Drawing for the job (mm, zero at the part's lowest x, y, z). A direction names the side the tool comes from. Give positions to 0.01 mm unless a question says otherwise; leave off trailing zeros. Order: outer loops, then holes, each group sorted by start corner. A loop starts at its lowest first (then second) coordinate and runs counter-clockwise, first axis right, second up. Notation, with made-up numbers: (16.5, 67) -> (47.5, 67) arc R19 cw to (47.5, 94) -> close; hole circle Ø5 at (-31.75, -21.5). An arc over 180 degrees is marked (long way). One line per item, written item: value. Start each with the question number.
(1) Saw through at B-B on y = 12.5. Give the cut face in (x, z).
(2) Which spindle directions (+Z, -Z, +X, -X, +Y, -Y) get a long thin tool onto all of the face, cutting with end or side? Do the marked faces 1 and 2. Say none if no direction does.
(3) Saw through at A-A on z = 2.4. Give the cut face in (x, y) (1 decimal).
(4) Probe line 1 (X direction, y = 4.5, z = 2.2); line 2 (Y direction, x = 1.65, z = 1.5) (1 decimal); line 3 (Y direction, x = 1.8, z = 1.6) (1 decimal). List the from-to ranges inside material, lowest first.
(5) Saw through at C-C on x = 2.75. Give the cut face in (y, z).
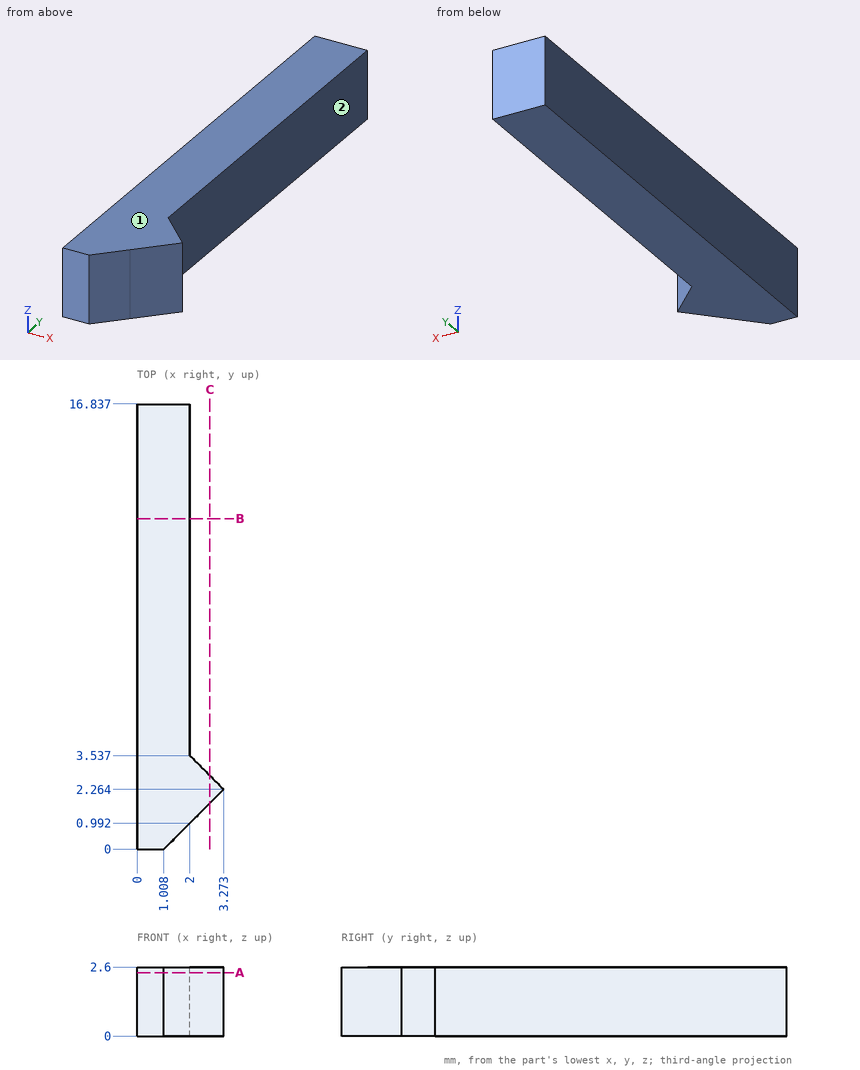
Results below:
1. outline: (0, 0) -> (2, 0) -> (2, 2.6) -> (0, 2.6) -> close
2. face 1: +Z, +X, -X, +Y, -Y
2. face 2: +Z, -Z, +X, +Y
3. outline: (0, 0) -> (1, 0) -> (2, 1) -> (3.3, 2.3) -> (2, 3.5) -> (2, 16.8) -> (0, 16.8) -> close
4. line 1: x = 0 to 2
4. line 2: y = 0.6 to 16.8
4. line 3: y = 0.8 to 16.8
5. outline: (1.74, 0) -> (2.79, 0) -> (2.79, 2.6) -> (1.74, 2.6) -> close
